Input: part model. Units: mm. Frame: model coordinates. Face numbers are marked on the shaded views. A direction names the side the tool comes from. Round coordinates to 2 decimals unless told otherwise and drop trailing zeros. Loops run counter-clockwise (first coordinate to the right, second up) from the corner with the lowest first, then second, coordinate; pieces in that order, holes last.
1) Section B-B, the plane x = 0. Return loops of the section in (y, z), and give its area (3 significant figures).
2) Access query for the marked faces 1, 2 and 3. Directions: +Z, -Z, +X, -X, +Y, -Y. A direction counts if a zero-diameter tool reaches every point of the face in a straight line with its end or side. Return the directions, or none.
3) First-contact query: pin 1 (1.5 mm diameter, centred on x = -12.5, y = -8, fed in from +Z); pin 2 (1 mm diameter, centred on x = -9, z = 1, fed in from -Y); pin 3 (1.6 mm diameter, centred on x = -12, z = 2.5, fed in from -Y); pin 4 (1.2 mm diameter, centred on y = -14, z = 2.5, fed in from -X). Flat tips, straight axial feed; report the tip coordinate or a pass-through.
4) Ray query, line 1 along X through (y, z) = (-10, 0.75); line 2 along Y through (x, z) = (0, 1.15); line 3 along Y through (x, z) = (-9, 1.5). Return the intervals inside material, ascending.
5) Draft query along X for the marked faces 4, 5 and 6. Return one class per face: pulls with the +X half, pulls with the -X half, needs draft (parallel to the pull), parting line crosses it, or undercut.
6) Section A-A, the plane y = 0. Return loops of the section in (x, z).
7) Section D-D, the plane y = -13. Return loops of the section in (x, z).
8) Section C-C, the plane x = -13.5. Return loops of the section in (y, z).
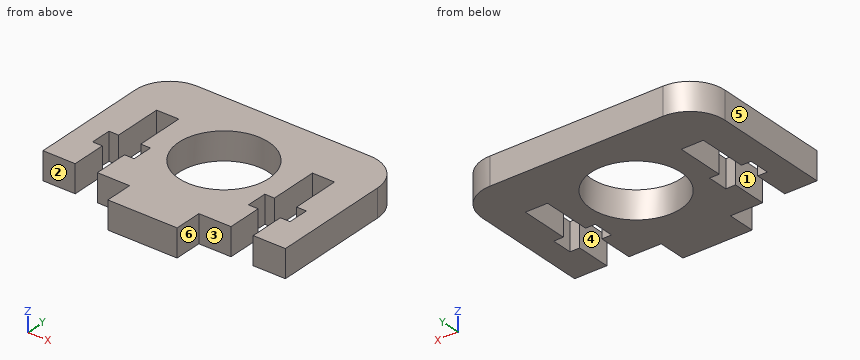
from build123d import *

# Parameters (mm, degrees)
SKETCH2_R           = 6.5
BOSS_EXTRUDE1_DEPTH = 4
CUT_EXTRUDE1_DEPTH  = 24.393375131
FILLET1_R           = 5


with BuildPart() as part:
    # Sketch2 → Boss-Extrude1 (new body)
    with BuildSketch(Plane.XY):
        Polygon((5, -11), (17.5, -11), (17.5, 11), (-17.5, 11), (-17.5, -11), (-5, -11), (-5, -15), (5, -15), align=None)
        Circle(SKETCH2_R, mode=Mode.SUBTRACT)
    extrude(amount=BOSS_EXTRUDE1_DEPTH)

    # Sketch3 → Cut-Extrude1 (cut, through all)
    with BuildSketch(Plane.XY.offset(4)):
        Polygon((12.85, -11), (12.85, -6), (14.25, -6), (14.25, -3), (12.85, -3), (12.85, 4), (9.65, 4), (9.65, -3), (8.25, -3), (8.25, -6), (9.65, -6), (9.65, -11), align=None)
        Polygon((-9.65, -11), (-12.85, -11), (-12.85, -6), (-14.25, -6), (-14.25, -3), (-12.85, -3), (-12.85, 4), (-9.65, 4), (-9.65, -3), (-8.25, -3), (-8.25, -6), (-9.65, -6), align=None)
    extrude(amount=-CUT_EXTRUDE1_DEPTH, mode=Mode.SUBTRACT)

    # Fillet1
    fillet1_edges = [part.edges().sort_by_distance(p)[0] for p in [
        (-17.5, 11, 2),
        (17.5, 11, 2),
    ]]
    fillet(fillet1_edges, radius=FILLET1_R)


solid = part.part
Final values:
1. outline: (-15, 0) - (-6.5, 0) - (-6.5, 4) - (-15, 4) - close; (6.5, 0) - (11, 0) - (11, 4) - (6.5, 4) - close
1. area: 52.0 mm2
2. face 1: +Z, -Z, -Y
2. face 2: +Z, -Z, -X, -Y
2. face 3: +Z, -Z, +X, -Y
3. pin 1: stops at z = 4
3. pin 2: stops at y = -11
3. pin 3: stops at y = 4
3. pin 4: stops at x = -5
4. line 1: x = -17.5 to -12.85, -9.65 to 9.65, 12.85 to 17.5
4. line 2: y = -15 to -6.5, 6.5 to 11
4. line 3: y = -11 to -6, -3 to 11
5. face 4: undercut
5. face 5: pulls with the -X half
5. face 6: pulls with the +X half
6. outline: (-17.5, 0) - (-12.85, 0) - (-12.85, 4) - (-17.5, 4) - close; (-9.65, 0) - (-6.5, 0) - (-6.5, 4) - (-9.65, 4) - close; (6.5, 0) - (9.65, 0) - (9.65, 4) - (6.5, 4) - close; (12.85, 0) - (17.5, 0) - (17.5, 4) - (12.85, 4) - close
7. outline: (-5, 0) - (5, 0) - (5, 4) - (-5, 4) - close
8. outline: (-11, 0) - (-6, 0) - (-6, 4) - (-11, 4) - close; (-3, 0) - (10.9, 0) - (10.9, 4) - (-3, 4) - close
